Read the model definition and answer for the solid it produces. Units are mm, in the model's axes. A direction names the side the tool comes from. Round coordinates to 2 decimals unless told otherwise and drop trailing zeros. Loops run counter-clockwise (first coordinate to the right, second up) from the corner with the lowest first, then second, coordinate; pieces in that order, holes last. Notation, with made-up numbers: (-34, -12.5) - (2, -12.5) arc R21 ccw to (2, 13.5) - close; hole circle Ø2 at (52, -7). An arc over 180 degrees is marked (long way). Answer as CSV lines item,"result".
Autodesk Inventor part; units mm, degrees
ref_plane "YZ Plane" through (0, 0, 0) normal (1, 0, 0) x (0, 1, 0)
ref_plane "XZ Plane" through (0, 0, 0) normal (0, 1, 0) x (-1, 0, 0)
ref_plane "XY Plane" through (0, 0, 0) normal (0, 0, 1) x (1, 0, 0)
sketch "Boceto1" plane through (0, 0, 0) normal (0, 1, 0) x (-1, 0, 0)
  circle A0 centre (0, 0) radius 10
  line L0 (7.0711, -7.0711) -> (0, -10)
  line L1 (10, 0) -> (7.0711, -7.0711)
  line L2 (0, -10) -> (-7.0711, -7.0711)
  line L3 (-10, 0) -> (-7.0711, -7.0711)
  line L4 (0, 10) -> (7.0711, 7.0711)
  line L5 (7.0711, 7.0711) -> (10, 0)
  line L6 (0, 0) -> (0, 10)
  line L7 (0, 10) -> (-7.0711, 7.0711)
  line L8 (-7.0711, 7.0711) -> (-10, 0)
  circle A1 centre (0, 0) radius 10
  line L9 (7.0711, -7.0711) -> (0, -10)
  line L10 (10, 0) -> (7.0711, -7.0711)
  line L11 (0, -10) -> (-7.0711, -7.0711)
  line L12 (-10, 0) -> (-7.0711, -7.0711)
  line L13 (0, 10) -> (7.0711, 7.0711)
  line L14 (7.0711, 7.0711) -> (10, 0)
  line L15 (0, 0) -> (0, 10)
  line L16 (-7.0711, 7.0711) -> (-10, 0)
  line L17 (0, 10) -> (-7.0711, 7.0711)
  dimension "d0" = 20
  dimension "d5" = 20
extrude "Extrusión1" add sketch "Boceto1" along normal blind 5 contours L1 L0 L2 L3 L8 L7 L4 L5
sketch "Boceto2" plane through (0, 5, 0) normal (0, 1, 0) x (1, 0, 0)
  circle A0 centre (0, 0) radius 9.2388
  line L0 (0, 10) -> (-7.0711, 7.0711)
extrude "Extrusión2" add sketch "Boceto2" along normal blind 20
sketch "Boceto3" plane through (0, 25, 0) normal (0, 1, 0) x (1, 0, 0)
  line L0 (7.0711, -7.0711) -> (8.5355, -3.5355)
  line L1 (8.5355, -3.5355) -> (10, 0)
  line L2 (10, 0) -> (8.5355, 3.5355)
  line L3 (8.5355, 3.5355) -> (7.0711, 7.0711)
  line L4 (7.0711, 7.0711) -> (3.5355, 8.5355)
  line L5 (3.5355, 8.5355) -> (0, 10)
  line L6 (0, -10) -> (3.5355, -8.5355)
  line L7 (3.5355, -8.5355) -> (7.0711, -7.0711)
  line L8 (0, -10) -> (7.0711, -7.0711)
  line L9 (7.0711, -7.0711) -> (10, 0)
  line L10 (10, 0) -> (7.0711, 7.0711)
  line L11 (10, 0) -> (7.0711, 7.0711)
  line L12 (7.0711, 7.0711) -> (0, 10)
  line L13 (0, 0) -> (0, 10)
  line L14 (-7.0711, -7.0711) -> (-8.5355, -3.5355)
  line L15 (-8.5355, -3.5355) -> (-10, 0)
  line L16 (-10, 0) -> (-8.5355, 3.5355)
  line L17 (-8.5355, 3.5355) -> (-7.0711, 7.0711)
  line L18 (-7.0711, 7.0711) -> (-3.5355, 8.5355)
  line L19 (-3.5355, 8.5355) -> (0, 10)
  line L20 (0, -10) -> (-3.5355, -8.5355)
  line L21 (-3.5355, -8.5355) -> (-7.0711, -7.0711)
  line L22 (0, -10) -> (-7.0711, -7.0711)
  line L23 (-7.0711, -7.0711) -> (-10, 0)
  line L24 (-10, 0) -> (-7.0711, 7.0711)
  line L25 (-10, 0) -> (-7.0711, 7.0711)
  line L26 (-7.0711, 7.0711) -> (0, 10)
extrude "Extrusión3" add sketch "Boceto3" along normal blind 7.5
sketch "Boceto4" plane through (0, 32.5, 0) normal (0, 1, 0) x (1, 0, 0)
  point P0 (0, 0)
  point P1 (0, 0)
hole "Agujero1" at (0, 32.5, 0) direction (0, -1, 0) diameter 15.1638 end through all
properties part number "TUBO_METALICO"
1) The mould has two halves that part along Z. Classify faces 6 (the face through (6.8, 25, 6.6)), 7 (the face through (7.402, 16.022, -1.644)), 8 (the face through (3.486, 2.465, 8.556)): pulls with the +Z half, pulls with the -Z half, needs draft (parallel to the pull), parting line crosses it, or undercut.
Entries:
face 6,"needs draft"
face 7,"undercut"
face 8,"pulls with the +Z half"
2) A cutting plane is placed at A-A, the plane x = -1.5. Determine the outline of the cut face in (y, z), plus the area to 3 significant figures.
Entries:
outline,"(0, -9.38) - (5, -9.38) - (5, -9.12) - (25, -9.12) - (25, -9.38) - (32.5, -9.38) - (32.5, -7.43) - (0, -7.43) - close; (0, 7.43) - (32.5, 7.43) - (32.5, 9.38) - (25, 9.38) - (25, 9.12) - (5, 9.12) - (5, 9.38) - (0, 9.38) - close"
area,"116 mm^2"
3) A cutting plane is placed at B-B, the plane z = 6. Determine the outline of the cut face in (x, y), plus the area to 3 significant figures.
Entries:
outline,"(-7.51, 0) - (-4.64, 0) - (-4.64, 32.5) - (-7.51, 32.5) - (-7.51, 25) - (-7.03, 25) - (-7.03, 5) - (-7.51, 5) - close; (4.64, 0) - (7.51, 0) - (7.51, 5) - (7.03, 5) - (7.03, 25) - (7.51, 25) - (7.51, 32.5) - (4.64, 32.5) - close"
area,"168 mm^2"
4) A tool of negligible diameter and unlimited length cuts with its end or side. For faces 1 (the face through (0, 25, 9.4)), 2 (the face through (0, 25, -9.4)), 3 (the face through (-6.6, 25, -6.8)), 4 (the face through (6.8, 25, -6.6)), 5 (the face through (-5.88, 5, -7.36)), from which of +Z, -Z, +X, -X, +Y, -Y can it reach the whole face along a straight path? Write none if from no direction.
Entries:
face 1,"+Z"
face 2,"-Z"
face 3,"-Z, -X"
face 4,"-Z, +X"
face 5,"none"
5) Each of these flat-tipped pins is pushed along its axis until it touches: P1, Ø1, axis at x = -4, y = 9.5, coming from the -Z side; P2, Ø5, axis at y = 26, z = 4.5, coming from the +X side; P3, Ø12, axis at y = 27.5, z = -7, coming from the -X side. Where does it stop, or does it pass through?
Entries:
P1,"stops at z = -8.55"
P2,"stops at x = 9.17"
P3,"stops at x = -9.59"
6) A cutting plane is placed at C-C, the plane y = 16.5. Determine the outline of the cut face in (x, z), plus the area to 3 significant figures.
Entries:
outline,"circle Ø18.48 at (0, 0); hole circle Ø15.16 at (0, 0)"
area,"87.6 mm^2"
7) Find the intervals of material crossed by line 1 (X direction, y = 20.5, z = 0); line 2 (Y direction, x = -5.5, z = -7.5), in increasing order.
Entries:
line 1,"x = -9.24 to -7.58, 7.58 to 9.24"
line 2,"y = 0 to 5, 25 to 32.5"
